```python
from build123d import *

# Parameters (mm, degrees)
BOSS_EXTRUDE4_DEPTH  = 1.5875
M3_CLEARANCE_HOLE3_D = 3
M3_CLEARANCE_HOLE1_D = 3.1
M3_CLEARANCE_HOLE4_D = 2.95
M3_CLEARANCE_HOLE2_D = 3.1
BOSS_EXTRUDE6_DEPTH  = 3.175
FILLET1_R            = 2
FILLET3_R            = 1
FILLET6_R            = 0.5
CUT_EXTRUDE4_DEPTH   = 10
SKETCH29_R           = 1.5
CUT_EXTRUDE5_DEPTH   = 10
SKETCH31_R           = 1.5
CUT_EXTRUDE7_DEPTH   = 10


with BuildPart() as part:
    # Sketch1 → Boss-Extrude4 (new, symmetric)
    with BuildSketch(Plane(origin=(0, 0, 0), x_dir=(1, 0, 0), z_dir=(0, 1, 0))):
        with BuildLine():
            Line((-62.799553621, 32.496136604), (-73.969425011, 32.691107434))
            Line((-73.969425011, 32.691107434), (-77.053684287, 35.88495141))
            ThreePointArc((-77.053684287, 35.88495141), (-84.36642289, 10.358894189), (-83.446216027, -16.178041625))
            Line((-83.446216027, -16.178041625), (-79.680911643, -13.825218315))
            Line((-79.680911643, -13.825218315), (-69.484649137, -16.179210996))
            Line((-69.484649137, -16.179210996), (-43.894490772, -57.132025032))
            Line((-43.894490772, -57.132025032), (-43.894490772, -64.826600275))
            Line((-43.894490772, -64.826600275), (-43.094490772, -64.826600275))
            Line((-43.094490772, -64.826600275), (-34, -64.826600275))
            Line((-34, -64.826600275), (-34, -62.55))
            Line((-34, -62.55), (-34, -61.55))
            Line((-34, -61.55), (-20, -61.55))
            Line((-20, -61.55), (-19.859459165, -62.55))
            Line((-19.859459165, -62.55), (19.859459165, -62.55))
            Line((19.859459165, -62.55), (20, -61.55))
            Line((20, -61.55), (34, -61.55))
            Line((34, -61.55), (34, -62.55))
            Line((34, -62.55), (34, -64.826600275))
            Line((34, -64.826600275), (43.094490772, -64.826600275))
            Line((43.094490772, -64.826600275), (43.894490772, -64.826600275))
            Line((43.894490772, -64.826600275), (43.894490772, -57.132025032))
            Line((43.894490772, -57.132025032), (69.484649137, -16.179210996))
            Line((69.484649137, -16.179210996), (79.680911643, -13.825218315))
            Line((79.680911643, -13.825218315), (83.446216027, -16.178041625))
            ThreePointArc((83.446216027, -16.178041625), (84.610662337, -8.126242604), (85, 0))
            ThreePointArc((85, 0), (82.98964744, 18.377116688), (77.053684287, 35.88495141))
            Line((77.053684287, 35.88495141), (73.969425011, 32.691107434))
            Line((73.969425011, 32.691107434), (62.799553621, 32.496136604))
            Line((62.799553621, 32.496136604), (30.284668021, 63.895396642))
            Line((30.284668021, 63.895396642), (30.089697191, 75.065268032))
            Line((30.089697191, 75.065268032), (33.173956467, 78.259112008))
            ThreePointArc((33.173956467, 78.259112008), (0, 85), (-33.173956467, 78.259112008))
            Line((-33.173956467, 78.259112008), (-30.089697191, 75.065268032))
            Line((-30.089697191, 75.065268032), (-30.284668021, 63.895396642))
            Line((-30.284668021, 63.895396642), (-62.799553621, 32.496136604))
        make_face()
    extrude(amount=BOSS_EXTRUDE4_DEPTH, both=True)

    # M3 Clearance Hole3 (through all)
    with Locations(Plane(origin=(0, -1.5875, 0), x_dir=(-1, 0, 0), z_dir=(0, -1, 0))):
        with Locations((36.5, -50), (36.5, -38), (-36.5, -50), (-36.5, -38)):
            Hole(M3_CLEARANCE_HOLE3_D / 2)

    # M3 Clearance Hole1 (through all)
    with Locations(Plane(origin=(0, 1.5875, 0), x_dir=(1, 0, 0), z_dir=(0, 1, 0))):
        with Locations((-78.542321426, -8.49139241), (78.542321426, -8.49139241), (74.155025063, 27.240269049), (-74.155025063, 27.240269049)):
            Hole(M3_CLEARANCE_HOLE1_D / 2)

    # M3 Clearance Hole4 (through all)
    with Locations(Plane(origin=(0, -1.5875, 0), x_dir=(-1, 0, 0), z_dir=(0, -1, 0))):
        with Locations((-67.099301622, -15.278865202), (-50.141885166, -42.416404279), (-61.062544382, 30.698137949), (-38.043670771, 52.927205804), (50.141885166, -42.416404279), (67.099301622, -15.278865202), (38.043670771, 52.927205804), (61.062544382, 30.698137949)):
            Hole(M3_CLEARANCE_HOLE4_D / 2)

    # M3 Clearance Hole2 (through all)
    with Locations(Plane(origin=(0, 1.5875, 0), x_dir=(1, 0, 0), z_dir=(0, 1, 0))):
        with Locations((27, 76.497766718), (-27, 76.497766718)):
            Hole(M3_CLEARANCE_HOLE2_D / 2)

    # Sketch22 → Boss-Extrude6 (add)
    with BuildSketch(Plane(origin=(0, 1.5875, 0), x_dir=(1, 0, 0), z_dir=(0, 1, 0))):
        Polygon((65.061950694, 32.535626892), (30.245177733, 66.157793715), (30.284668021, 63.895396642), (62.799553621, 32.496136604), align=None)
        Polygon((-30.284668021, 63.895396642), (-30.245177733, 66.157793715), (-65.061950694, 32.535626892), (-62.799553621, 32.496136604), align=None)
        Polygon((43.894490772, -60.151352895), (71.689396914, -15.670204865), (69.484649137, -16.179210996), (43.894490772, -57.132025032), align=None)
        Polygon((-69.484649137, -16.179210996), (-71.689396914, -15.670204865), (-43.894490772, -60.151352895), (-43.894490772, -57.132025032), align=None)
    extrude(amount=-BOSS_EXTRUDE6_DEPTH)

    # Fillet1
    fillet1_edges = [part.edges().sort_by_distance(p)[0] for p in [
        (-30.245177733, 0.79375, -66.157793715),
        (-65.061950694, 0.79375, -32.535626892),
        (-71.689396914, 0.79375, 15.670204865),
        (-43.894490772, 0.79375, 60.151352895),
        (43.894490772, -0.79375, 60.151352895),
        (71.689396914, -0.79375, 15.670204865),
        (65.061950694, 0.79375, -32.535626892),
        (30.245177733, -0.79375, -66.157793715),
        (30.089697191, -0.79375, -75.065268032),
        (73.969425011, -0.79375, -32.691107434),
        (79.680911643, -0.79375, 13.825218315),
        (-79.680911643, -0.79375, 13.825218315),
        (-73.969425011, -0.79375, -32.691107434),
        (-30.089697191, -0.79375, -75.065268032),
    ]]
    fillet(fillet1_edges, radius=FILLET1_R)

    # Fillet3
    fillet3_edges = [part.edges().sort_by_distance(p)[0] for p in [
        (33.173956467, -0.79375, -78.259112008),
        (77.053684287, 0.79375, -35.88495141),
        (83.446216027, -0.79375, 16.178041625),
        (43.894490772, -0.79375, 64.826600275),
        (34, 0.79375, 64.826600275),
        (34, -0.79375, 61.55),
        (-34, -0.79375, 61.55),
        (-34, 0.79375, 64.826600275),
        (-43.894490772, -0.79375, 64.826600275),
        (-83.446216027, -0.79375, 16.178041625),
        (-77.053684287, -0.79375, -35.88495141),
        (-33.173956467, -0.79375, -78.259112008),
    ]]
    fillet(fillet3_edges, radius=FILLET3_R - 0.0001)  # a hair under: the kernel refuses the full size

    # Fillet6
    fillet6_edges = [part.edges().sort_by_distance(p)[0] for p in [
        (20, -0.79375, 61.55),
        (19.859459165, -0.79375, 62.55),
        (-19.859459165, 0.79375, 62.55),
        (-20, 0.79375, 61.55),
    ]]
    fillet(fillet6_edges, radius=FILLET6_R)

    # Sketch28 → Cut-Extrude4 (cut)
    with BuildSketch(Plane(origin=(0, 1.5875, 0), x_dir=(1, 0, 0), z_dir=(0, 1, 0))):
        with BuildLine():
            Line((-26.25, -12.55), (-26.25, -62.55))
            Line((-26.25, -62.55), (26.25, -62.55))
            Line((26.25, -62.55), (26.25, -12.55))
            Line((26.25, -12.55), (21.2, -12.55))
            Line((21.2, -12.55), (21.2, -4.5))
            Line((21.2, -4.5), (4.195235393, -4.5))
            ThreePointArc((4.195235393, -4.5), (0, -0.5), (-4.195235393, -4.5))
            Line((-4.195235393, -4.5), (-21.2, -4.5))
            Line((-21.2, -4.5), (-21.2, -12.55))
            Line((-21.2, -12.55), (-26.25, -12.55))
        make_face()
    extrude(amount=-CUT_EXTRUDE4_DEPTH, mode=Mode.SUBTRACT)

    # Sketch29 → Cut-Extrude5 (cut)
    with BuildSketch(Plane(origin=(0, 1.5875, 0), x_dir=(1, 0, 0), z_dir=(0, 1, 0))):
        with Locations(Location((30.25, -56.55, 0), (0, 0, 270))):
            Circle(SKETCH29_R)
        with Locations(Location((-30.25, -56.55, 0), (0, 0, 270))):
            Circle(SKETCH29_R)
    extrude(amount=-CUT_EXTRUDE5_DEPTH, mode=Mode.SUBTRACT)

    # Sketch31 → Cut-Extrude7 (cut)
    with BuildSketch(Plane(origin=(0, 1.5875, 0), x_dir=(1, 0, 0), z_dir=(0, 1, 0))):
        with Locations(Location((-26, -9.55, 0), (0, 0, 270))):
            Circle(SKETCH31_R)
        with Locations(Location((26, -9.55, 0), (0, 0, 270))):
            Circle(SKETCH31_R)
    extrude(amount=-CUT_EXTRUDE7_DEPTH, mode=Mode.SUBTRACT)


solid = part.part
```
Work out the finished part from the listing and answer in its coordinate system (mm). Round coordinates to 2 decimals unless told otherwise and drop trailing zeros. Write each loop counter-clockwise with the first axis right and the second up, starting at its lowest first coordinate (ties: lowest second). Pieces come first, ordered by that corner, then holes. Notation, with made-up numbers: (22, -32.75) - (28, -32.75) arc R10 cw to (28, -14.75) - close; hole circle Ø11 at (58, -32). An arc over 180 degrees is marked (long way). Return JSON: item names as keys, results as strings. Group by question number.
Q1. Each of these flat-tipped pins is pushed along its axis until it touches: pin 1 Ø1 at (y, z) = (0.5, 45.5) entering from -X; pin 2 Ø1.6 at (x, y) = (-29, -0.5) entering from +Z; pin 3 Ø1 at (y, z) = (0.5, 9.5) entering from +X. Where does it stop, or does it pass through?
Q2. The part is cut by section C-C on y = 0.75. Count the separate pieces of the cut face and the enclosed holes in it, then the cut area to 3 significant figures.
Q3. The mould has two halves that part along X. Classify faces 1 (the cylindrical face through (0.1, 0, 0.5)), 2 (the cylindrical face through (84.41, 0.02, -10.01)), 3 (the flat face through (-57.91, 0.02, 37.72)): released by +X, released by -X, zero draft, split by the parting line, or undercut.
Q4. Find the intervals of material crossed by L1, parallel to Z at x = 35.5, y = 0.05; L2, parallel to X at y = -0.15, z = 39; L3, parallel to X at y = 0.55, z = 38, in increasing order.
Q5. The part is cut by section B-B on x = 0. Write down the section's boundary in (y, z), then the cut area to 3 significant figures.
Q6. The part is cut by section A-A on z = 2.5. Write down the section's boundary in (x, y).
Solved:
{
 "1": {"pin 1": "x = -53.36", "pin 2": "z = 61.55", "pin 3": "x = 84.52"},
 "2": {"separate pieces": "1", "enclosed holes": "22", "area": "14,500 mm²"},
 "3": {"face 1": "undercut", "face 2": "released by +X", "face 3": "released by -X"},
 "4": {"L1": "-61.08 to 36.88, 39.12 to 48.88, 51.12 to 64.83", "L2": "-57.11 to -37.62, -35.38 to -26.25, 26.25 to 35.38, 37.62 to 57.11", "L3": "-57.74 to -38, -35 to -26.25, 26.25 to 35, 38 to 57.74"},
 "5": {"outline": "(-1.59, -85) - (1.59, -85) - (1.59, 0.5) - (-1.59, 0.5) - close", "area": "271 mm²"},
 "6": {"outline": "(-84.96, -1.59) - (-3.58, -1.59) - (-3.58, 1.59) - (-84.96, 1.59) - close; (3.58, -1.59) - (84.96, -1.59) - (84.96, 1.59) - (3.58, 1.59) - close"}
}
